Could you check a few things on this model? Use its own coordinates, in mm. Face numbers are marked on the shaded views. Give positions to 0.01 mm unless a question says otherwise; leave off trailing zeros. Write each loop counter-clockwise with the first axis right and the second up, starting at its lowest first coordinate (ties: lowest second). Pieces come first, ordered by that corner, then holes. Notation, with made-up numbers: (-8.5, 78.5) - (10.5, 78.5) arc R33 cw to (10.5, 110.5) - close; hole circle Ø7 at (18, -25). An arc over 180 degrees is marked (long way). Use one line per item in the form item = value.
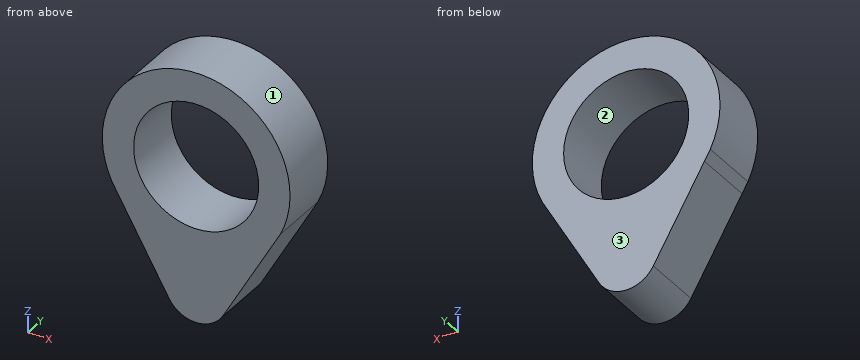
```python
from build123d import *

# Parameters (mm, degrees)
F0_R     = 12.7
F1_DEPTH = 12.7


with BuildPart() as f1:
    # F0 (on Front) → F1 (new body)
    with BuildSketch(Plane.XZ):
        with BuildLine():
            Line((-15.887629, -10.51122), (-5.504633, -28.565677))
            ThreePointArc((-5.504633, -28.565677), (0, -31.75), (5.504633, -28.565677))
            Line((5.504633, -28.565677), (17.075518, -8.445661))
            ThreePointArc((17.075518, -8.445661), (0, 19.05), (-17.075518, -8.445661))
            Line((-17.075518, -8.445661), (-15.887629, -10.51122))
        make_face()
        Circle(F0_R, mode=Mode.SUBTRACT)
    extrude(amount=F1_DEPTH)


solid = f1.part
```
1. Imagine slicing it at D-D, the plane z = -16.5. List the corners of the cut face in (x, y) for me.
Response values:
outline = (-12.44, -12.7) - (12.44, -12.7) - (12.44, 0) - (-12.44, 0) - close
2. If I drill on line 1 (Z direction, x = 4, y = -3.25); line 2 (Z direction, x = 9, y = -6.75); line 3 (X direction, y = -10.5, z = 3.5), over which ranges is the centre line in solid material (lowest first)? Write a range as from..to.
Response values:
line_1 = -30.33..-12.05, 12.05..18.63
line_2 = -22.49..-8.96, 8.96..16.79
line_3 = -18.73..-12.21, 12.21..18.73
3. Imagine slicing it at C-C, the plane y = -8.25. List the corners of the cut face in (x, z) for me, and give its area (3 significant figures).
Response values:
outline = (-17.08, -8.45) - (-5.5, -28.57) arc R6.35 ccw to (5.5, -28.57) - (17.08, -8.45) arc R19.05 ccw (long way) to start; hole circle Ø25.4 at (0, 0)
area = 853 mm²
4. For pin 1 (5 mm diameter, centred on x = -13, y = -3, fed in from +Z); pin 2 (1 mm diameter, centred on x = 5, y = -10.5, fed in from +Z); pin 3 (6 mm diameter, centred on y = -3, z = -14, fed in from +X), each with a flat end and sliding along its axis, tell me the tip position at first contact or that it passes through.
Response values:
pin_1 = 15.9
pin_2 = 18.51
pin_3 = 15.61
5. Imagine slicing it at A-A, the plane x = 0. List the corners of the cut face in (y, z) for me.
Response values:
outline = (-12.7, -31.75) - (0, -31.75) - (0, -12.7) - (-12.7, -12.7) - close; (-12.7, 12.7) - (0, 12.7) - (0, 19.05) - (-12.7, 19.05) - close
6. If we mould it in two halves opening along X, with no side actions, what happens to the marked faces 1, 2 and 3? For each: pulls with the +X half, pulls with the -X half, needs draft (parallel to the pull), parting line crosses it, or undercut.
Response values:
face_1 = parting line crosses it
face_2 = undercut
face_3 = needs draft
7. Imagine slicing it at B-B, the plane z = 0. List the corners of the cut face in (x, y) for me, and give its area (3 significant figures).
Response values:
outline = (-19.05, -12.7) - (-12.7, -12.7) - (-12.7, 0) - (-19.05, 0) - close; (12.7, -12.7) - (19.05, -12.7) - (19.05, 0) - (12.7, 0) - close
area = 161 mm²
